from build123d import *

# Parameters (mm, degrees)
CHAMFER1_SIZE = 0.2


with BuildPart() as part:
    # Sketch1 → Revolve1 (revolve)
    with BuildSketch(Plane.XY, mode=Mode.PRIVATE) as revolve1_sk:
        Polygon((0, 13.5), (2, 13.5), (2, 15), (20, 15), (20, 16.05), (21.2, 16.05), (21.2, 15), (23, 15), (23, 30), (0, 30), align=None)
    revolve(revolve1_sk.sketch.rotate(Axis((0, 0, 0), (1, 0, 0)), 90), axis=Axis((0, 0, 0), (1, 0, 0)))

    # Chamfer1
    chamfer1_edges = [part.edges().sort_by_distance(p)[0] for p in [
        (2, 0, -13.5),
        (0, 0, -13.5),
        (0, 0, -30),
        (23, 0, -30),
        (23, 0, -15),
    ]]
    chamfer(chamfer1_edges, length=CHAMFER1_SIZE)


solid = part.part
For this review, take the finished solid that the model builds, in its own axes (mm). A direction names the side the tool comes from. Round coordinates to 2 decimals unless told otherwise and drop trailing zeros. Write each loop counter-clockwise with the first axis right and the second up, starting at its lowest first coordinate (ties: lowest second). Pieces come first, ordered by that corner, then holes. Notation, with made-up numbers: (-39.75, 83.25) -> (-20.75, 83.25) arc R21 cw to (-20.75, 120.25) -> close; hole circle Ø3 at (6.25, 65.25). An arc over 180 degrees is marked (long way). Put each result on its own line as item: value.
Q1. Machinability: for faces 4 (the cylindrical face through (20.61, -4.82, 15.31)), 5 (the flat face through (0, 13, 6)), 6 (the flat face through (2, 12, -7)), which of the approach directions +Z, -Z, +X, -X, +Y, -Y give a long, thin tool a straight path to every point of the face, cutting with its end or side? Answer none if there is none.
Determined:
face 4: none
face 5: +Z, -Z, -X, +Y, -Y
face 6: +X
Q2. The part is to be moulded in two halves that separate along Y. For faces 1 (the cylindrical face through (1.01, 13.18, -2.93)), 2 (the cylindrical face through (11.342, -25.296, 16.128)), 3 (the flat face through (23, -7, 14)), say which applies: released by +Y, released by -Y, zero draft, split by the parting line, or undercut.
Determined:
face 1: undercut
face 2: split by the parting line
face 3: zero draft
Q3. Clearance check with flat-ended pins moving along their axes: pin 1 Ø6 at (x, y) = (7.5, -21) entering from +Z; pin 2 Ø16 at (y, z) = (2, -1.5) entering from -X; pin 3 Ø6 at (x, y) = (16, -10.5) entering from -Z; pin 4 Ø1 at (x, z) = (12.5, 10.5) entering from -Y. State where each tip first meets the part, or that it passes through.
Determined:
pin 1: stops at z = 24
pin 2: passes through
pin 3: stops at z = -29.05
pin 4: stops at y = -28.28
Q4. Consider section C-C on x = 3. State the section outline as (y, z) points, and give its area (3 significant figures).
Determined:
outline: circle Ø60 at (0, 0); hole circle Ø30 at (0, 0)
area: 2,120 mm^2
Q5. To check wall thickness, follow L1, parallel to X at y = 9, z = -13; L2, parallel to Y at x = 9.5, z = 0.5; L3, parallel to Y at x = 4.75, z = 13. State the ranges of each line that lie inside material, in increasing order. Write a range as [from, to].
Determined:
L1: x = [0, 20], [21.2, 23]
L2: y = [-30, -14.99], [14.99, 30]
L3: y = [-27.04, -7.48], [7.48, 27.04]
